Design review of the part built by this model. Coordinates are the model's own, in mm. A direction names the side the tool comes from. Give positions to 0.01 mm unless a question says otherwise; leave off trailing zeros. Loops run counter-clockwise (first coordinate to the right, second up) from the corner with the lowest first, then second, coordinate; pieces in that order, holes last. Notation, with made-up numbers: (-2.75, -20) -> (49.25, -20) arc R12 ccw to (49.25, 2) -> close; hole circle Ø7 at (88.25, 2.5). An arc over 180 degrees is marked (long way). Use CSV: the item, a comma, the result in double quotes. Start each with the question number.
Item 1: We need section A-A (y = 0). State the section outline as (x, z) points, plus the area to 3 significant figures.
Item 2: We need section C-C (z = 15.5). State the section outline as (x, y) points.
Item 3: Wall thickness on line 1 along Y through (x, z) = (0, 57.5); line 2 along Y through (x, z) = (0, 16.5); line 3 along X through (y, z) = (-2, 41.5): over which ranges is each line inside the solid? List them lowest first. Write a range as from..to.
Item 4: Clearance check with flat-ended pins moving along their axes: pin 1 (1.5 mm diameter, centred on y = 6, z = 14, fed in from +X); pin 2 (4.5 mm diameter, centred on x = 2.5, y = 3, fed in from +Z); pin 3 (8 mm diameter, centred on y = 6, z = 42, fed in from -X). State where each tip first meets the part, or that it passes through.
Item 5: The part is to be moulded in two halves that separate along X. For faces 1 (the face through (-2.17, -9.76, 34.51)), 2 (the face through (4, 5, 0)), 3 (the face through (-6.094, 0.268, 12.325)), say which applies: +X half, -X half, draft (parallel to the pull), parting line (faces both ways), or undercut.
Item 6: For faces 4 (the face through (7, 4, 70)), 5 (the face through (-7.593, 0.334, 47.815)), list the 3-axis set-ups (+Z, -Z, +X, -X, +Y, -Y) from which the entire face can be reached by the end or side of a thin tool; tool diameter is ignored.
Item 7: We need section D-D (z = 65.5). State the section outline as (x, y) points, plus the area to 3 significant figures.
from build123d import *

# Parameters (mm, degrees)
SKETCH2_R           = 10
SKETCH2_R_2         = 6.1
BOSS_EXTRUDE1_DEPTH = 25
SKETCH3_R           = 10
BOSS_EXTRUDE2_DEPTH = 45
SKETCH4_R           = 7.6
CUT_EXTRUDE1_DEPTH  = 45


with BuildPart() as part:
    # Sketch2 → Boss-Extrude1 (new body)
    with BuildSketch(Plane.XY):
        Circle(SKETCH2_R)
        Circle(SKETCH2_R_2, mode=Mode.SUBTRACT)
    extrude(amount=BOSS_EXTRUDE1_DEPTH)

    # Sketch3 → Boss-Extrude2 (add)
    with BuildSketch(Plane.XY.offset(25)):
        Circle(SKETCH3_R)
    extrude(amount=BOSS_EXTRUDE2_DEPTH)

    # Sketch4 → Cut-Extrude1 (cut)
    with BuildSketch(Plane.XY.offset(70)):
        Circle(SKETCH4_R)
    extrude(amount=-CUT_EXTRUDE1_DEPTH, mode=Mode.SUBTRACT)


solid = part.part
Results found:
1,outline,"(-10, 0) -> (-6.1, 0) -> (-6.1, 25) -> (-7.6, 25) -> (-7.6, 70) -> (-10, 70) -> close; (6.1, 0) -> (10, 0) -> (10, 70) -> (7.6, 70) -> (7.6, 25) -> (6.1, 25) -> close"
1,area,"411 mm²"
2,outline,"circle Ø20 at (0, 0); hole circle Ø12.2 at (0, 0)"
3,line 1,"-10..-7.6, 7.6..10"
3,line 2,"-10..-6.1, 6.1..10"
3,line 3,"-9.8..-7.33, 7.33..9.8"
4,pin 1,"x = 8.51"
4,pin 2,"z = 25"
4,pin 3,"x = -9.8"
5,face 1,"parting line"
5,face 2,"draft"
5,face 3,"undercut"
6,face 4,"+Z, +X, -X, +Y, -Y"
6,face 5,"+Z"
7,outline,"circle Ø20 at (0, 0); hole circle Ø15.2 at (0, 0)"
7,area,"133 mm²"
